```python
from build123d import *

# Parameters (mm, degrees)
F3_D     = 3.2
F3_DEPTH = 10
F3_TIP   = 0.9613769904
F4_SIZE  = 0.5


with BuildPart() as f1:
    # F0 (on Front) → F1 (revolve)
    with BuildSketch(Plane.XZ):
        Polygon((0, 7.5), (0, 0), (50, 0), (55.1, 0), (55.1, 4), (50, 4), (50, 7.5), align=None)
    revolve(axis=Axis((25, 0, 0), (1, 0, 0)))

    # F3
    with Locations(Plane.YZ.offset(55.1)):
        with Locations((0, 0)):
            Hole(F3_D / 2, depth=F3_DEPTH)
            with Locations((0, 0, -(F3_DEPTH + F3_TIP / 2))):  # 118° drill point
                Cone(0, F3_D / 2, F3_TIP, mode=Mode.SUBTRACT)

    # F4
    f4_edges = [f1.edges().sort_by_distance(p)[0] for p in [
        (50, 0, -7.5),
        (0, 0, -7.5),
        (25, 0, 7.5),
        (55.1, 0, -4),
        (55.1, -1.6, 0),
    ]]
    chamfer(f4_edges, length=F4_SIZE)


solid = f1.part
```
Design review of the part built by this model. Coordinates are the model's own, in mm. A direction names the side the tool comes from. Coordinates: 2 decimals unless noted, no trailing zeros. Loops run counter-clockwise (first coordinate to the right, second up) from the corner with the lowest first, then second, coordinate; pieces in that order, holes last. Notation, with made-up numbers: M -26.75,79 L 30.25,79 A17 ccw 30.25,89 Z; hole C -25.75,-13.5 d6. An arc over 180 degrees is marked long. One line per question, with ' | ' between items.
(1) For pin 1 Ø4 at (y, z) = (-2.5, 3) entering from +X; pin 2 Ø4 at (x, z) = (21.5, 5.5) entering from +Y; pin 3 Ø1 at (x, z) = (17.5, -5) entering from +Y; pin 4 Ø3 at (y, z) = (0, 0) entering from +X, all flat-tipped, find the tip position at first contact; note any pin that passes through.
Filled in:
pin 1: stops at x = 55.1 | pin 2: stops at y = 6.63 | pin 3: stops at y = 6 | pin 4: stops at x = 45.04
(2) Wall thickness on probe 1 along Z at (x, y) = (48.5, 0); probe 2 along Z at (x, y) = (51.25, 0): over which ranges is each line inside the solid? List them lowest first.
Filled in:
probe 1: z = -7.5 to -1.6, 1.6 to 7.5 | probe 2: z = -4 to -1.6, 1.6 to 4
(3) We need section A-A (x = 40). Give the boundary of the cut face in (y, z), and give its area (3 significant figures).
Filled in:
outline: C 0,0 d15 | area: 177 mm^2
(4) Machinability: for faces 4 (the face through (52.268, 3.905, -0.867)), 5 (the face through (0, 0, 0)), which of the approach directions +Z, -Z, +X, -X, +Y, -Y give a long, thin tool a straight path to every point of the face, cutting with its end or side? Answer none if there is none.
Filled in:
face 4: +X | face 5: +Z, -Z, -X, +Y, -Y
(5) Draft analysis for pull direction Z (two halves, no side actions). For faces 1 (the face through (24.657, -0.33, -7.493)), 2 (the face through (49.78, 1.27, -0.97)), 3 (the face through (50, 3, -3)), state which applies: released by +Z, released by -Z, zero draft, split by the parting line, or undercut.
Filled in:
face 1: split by the parting line | face 2: undercut | face 3: zero draft
